Input: part model. Units: mm. Frame: model coordinates. A direction names the side the tool comes from. Round coordinates to 2 decimals unless told otherwise and drop trailing zeros. Loops run counter-clockwise (first coordinate to the right, second up) from the corner with the lowest first, then second, coordinate; pieces in that order, holes last. Notation, with made-up numbers: M 22,12.25 L 66,12.25 A37 cw 66,50.25 Z; hole C -28,49 d7. An arc over 180 degrees is marked long. Return JSON: item names as keys, results as strings. Group by question number.
1) Section B-B (x = 3.5). Output: boundary loops of the cut face in (y, z).
2) Material intervals for line 1 (Y direction, x = -5.25, z = 0); line 2 (Y direction, x = 12.5, z = 0); line 3 (Z direction, x = 14.25, y = 1), sorted ascending. Write a range as from..to.
3) Section C-C (y = 68.5). Output: boundary loops of the cut face in (x, z), plus the area to 3 significant figures.
4) Access query for faces 1 (the face through (9.86, 38.668, 5.077)), 2 (the face through (-3, -17, -1)), 3 (the face through (-3.04, 1.21, -87.49)). Directions: +Z, -Z, +X, -X, +Y, -Y. A direction counts if a zero-diameter tool reaches every point of the face in a straight line with its end or side. Return the directions, or none.
5) Mould query, pull axis Y, two halves, no side actions, for faces 4 (the face through (-3, -0.1, 92.5)), 5 (the face through (20, 29.1, -26.3)), 6 (the face through (-2.96, 7.81, 1.73)). Classes: +Y half, -Y half, draft (parallel to the pull), parting line (faces both ways), or undercut.
6) Contact query for flat-ended pins moving along their axis: P1, Ø4, axis at y = 38.5, z = 2.5, coming from the -X side; P2, Ø2, axis at y = 30.5, z = 10, coming from the +X side; P3, Ø6, axis at x = -2, y = 23.5, coming from the +Z side; P4, Ø6, axis at y = 75.78, z = -43.75, coming from the -X side. Output: stop coordinate, or through.
7) Section D-D (y = 0). Count the separate pieces of the cut face and the enclosed holes in it, plus the area to 3 significant figures.
from build123d import *

# Parameters (mm, degrees)
SKETCH1_W           = 6
SKETCH1_H           = 87.5
SKETCH3_R           = 8
CUT_EXTRUDE2_DEPTH  = 30
SKETCH4_R           = 5
BOSS_EXTRUDE1_DEPTH = 6
CIRPATTERN2_COUNT   = 3
SKETCH6_R           = 2.5
CUT_EXTRUDE3_DEPTH  = 6
CIRPATTERN3_COUNT   = 3
SKETCH8_R           = 17.5
SKETCH8_R_2         = 10
BOSS_EXTRUDE2_DEPTH = 15
SKETCH10_R          = 44
SKETCH10_R_2        = 39
BOSS_EXTRUDE3_DEPTH = 20
SKETCH11_R          = 81.5
CUT_EXTRUDE4_DEPTH  = 3
SKETCH12_R          = 15
SKETCH12_R_2        = 8
BOSS_EXTRUDE4_DEPTH = 3


with BuildPart() as part:
    # Sketch1 → Revolve1 (revolve)
    with BuildSketch(Plane(origin=(0, 0, 0), x_dir=(-1, 0, 0), z_dir=(0, 1, 0)), mode=Mode.PRIVATE) as revolve1_sk:
        with Locations((3, 43.75)):
            Rectangle(SKETCH1_W, SKETCH1_H)
    revolve(revolve1_sk.sketch.rotate(Axis((38.11091851, 0, 0), (-1, 0, 0)), 180), axis=Axis((38.11091851, 0, 0), (-1, 0, 0)))

    # Sketch3 → Cut-Extrude2 (cut)
    with BuildSketch(Plane.YZ):
        with Locations(Location((0, 0, 0), (0, 0, 270))):
            Circle(SKETCH3_R)
    extrude(amount=-CUT_EXTRUDE2_DEPTH, mode=Mode.SUBTRACT)

    # Sketch4 → Boss-Extrude1 (add)
    with BuildSketch(Plane(origin=(-6, 0, 0), x_dir=(0, -1, 0), z_dir=(-1, 0, 0))):
        with Locations((0, 87.5)):
            Circle(SKETCH4_R)
    boss_extrude1 = extrude(amount=-BOSS_EXTRUDE1_DEPTH)

    # CirPattern2: Boss-Extrude1 ×3 about axis
    cirpattern2_axis = Axis((0, 0, 0), (1, 0, 0))
    for i in range(1, CIRPATTERN2_COUNT):
        add(boss_extrude1.rotate(cirpattern2_axis, i * 360 / CIRPATTERN2_COUNT))

    # Sketch6 → Cut-Extrude3 (cut)
    with BuildSketch(Plane(origin=(-6, 0, 0), x_dir=(0, -1, 0), z_dir=(-1, 0, 0))):
        with Locations(Location((0, 87.5, 0), (0, 0, 90))):
            Circle(SKETCH6_R)
    cut_extrude3 = extrude(amount=-CUT_EXTRUDE3_DEPTH, mode=Mode.SUBTRACT)

    # CirPattern3: Cut-Extrude3 ×3 about axis
    cirpattern3_axis = Axis((0, 0, 0), (1, 0, 0))
    for i in range(1, CIRPATTERN3_COUNT):
        add(cut_extrude3.rotate(cirpattern3_axis, i * 360 / CIRPATTERN3_COUNT), mode=Mode.SUBTRACT)

    # Sketch8 → Boss-Extrude2 (add)
    with BuildSketch(Plane.YZ):
        with Locations(Location((0, 0, 0), (0, 0, 90))):
            Circle(SKETCH8_R)
        with Locations(Location((0, 0, 0), (0, 0, 270))):
            Circle(SKETCH8_R_2, mode=Mode.SUBTRACT)
    extrude(amount=BOSS_EXTRUDE2_DEPTH)

    # Sketch10 → Boss-Extrude3 (add)
    with BuildSketch(Plane.YZ):
        with Locations(Location((0, 0, 0), (0, 0, 90))):
            Circle(SKETCH10_R)
        with Locations(Location((0, 0, 0), (0, 0, 270))):
            Circle(SKETCH10_R_2, mode=Mode.SUBTRACT)
    extrude(amount=BOSS_EXTRUDE3_DEPTH)

    # Sketch11 → Cut-Extrude4 (cut)
    with BuildSketch(Plane(origin=(-6, 0, 0), x_dir=(0, -1, 0), z_dir=(-1, 0, 0))):
        with Locations(Location((0, 0, 0), (0, 0, 90))):
            Circle(SKETCH11_R)
    extrude(amount=-CUT_EXTRUDE4_DEPTH, mode=Mode.SUBTRACT)

    # Sketch12 → Boss-Extrude4 (add)
    with BuildSketch(Plane(origin=(-3, 0, 0), x_dir=(0, -1, 0), z_dir=(-1, 0, 0))):
        with Locations(Location((0, 0, 0), (0, 0, 270))):
            Circle(SKETCH12_R)
        with Locations(Location((0, 0, 0), (0, 0, 270))):
            Circle(SKETCH12_R_2, mode=Mode.SUBTRACT)
    extrude(amount=BOSS_EXTRUDE4_DEPTH)


solid = part.part
Returned:
{
 "1": {"outline": "C 0,0 d88; C 0,0 d35; hole C 0,0 d78; hole C 0,0 d20"},
 "2": {"line 1": "y = -87.5..-81.5, -15..-8, 8..15, 81.5..87.5", "line 2": "y = -44..-39, -17.5..-10, 10..17.5, 39..44", "line 3": "z = -43.99..-38.99, -17.47..-9.95, 9.95..17.47, 38.99..43.99"},
 "3": {"outline": "M -6,-54.44 L 0,-54.44 L 0,54.44 L -6,54.44 L -6,44.16 L -3,44.16 L -3,-44.16 L -6,-44.16 Z", "area": "388 mm^2"},
 "4": {"face 1": "+X", "face 2": "-X", "face 3": "-Z, +X, -X"},
 "5": {"face 4": "parting line", "face 5": "draft", "face 6": "undercut"},
 "6": {"P1": "stops at x = -3", "P2": "stops at x = 0", "P3": "stops at z = 85.06", "P4": "stops at x = -6"},
 "7": {"separate pieces": "3", "enclosed holes": "0", "area": "980 mm^2"}
}
